Here's how the part is built. I have some questions about the finished solid (model axes, mm). Round coordinates to 2 decimals unless told otherwise and drop trailing zeros. Write each loop counter-clockwise with the first axis right and the second up, starting at its lowest first coordinate (ties: lowest second). Pieces come first, ordered by that corner, then holes. Notation, with made-up numbers: M 59,-8 L 108,-8 A25 cw 108,14 Z; hole C 7,67 d4. An arc over 180 degrees is marked long. Write item = value, one per line. Start each with the question number.
(1) I want a section at B-B (x = 63.5). List the corners of the cut face in (y, z) for me.
(2) Will these pins go through, and if not, where does the flat tip stop? pin 1 Ø2.5 at (x, z) = (142.5, -20) entering from +Y; pin 2 Ø1.2 at (x, y) = (-124, 1) entering from -Z.
(3) I want a section at C-C (y = 3.2). Give the number of separate pieces and of enclosed holes in the cut face, and give its area (3 significant figures).
(4) I need wall thicknesses on line 1 along X through (y, z) = (2.65, -60); line 2 along X through (y, z) = (1.3, 33); line 3 along X through (y, z) = (1.7, 187). Which ranges of each line are inside material? Lowest first, please.
(5) I want a section at A-A (x = -48). List the corners of the cut face in (y, z) for me.
```python
from build123d import *

# Parameters (mm, degrees)
SKETCH_1_W          = 300
SKETCH_1_H          = 500
EXTRUDE_1_DEPTH     = 4
SKETCH_2_R          = 2.5
CUT_EXTRUDE_5_DEPTH = 292.575033225
SKETCH_4_R          = 2
SKETCH_4_W          = 42
SKETCH_4_H          = 25
CUT_EXTRUDE_4_DEPTH = 292.575033225
SKETCH_5_R          = 2
CUT_EXTRUDE_6_DEPTH = 10
SKETCH_3_R          = 2
CUT_EXTRUDE_2_DEPTH = 292.575033225
CHAMFER_1_SIZE      = 2


with BuildPart() as part:
    # 草图1 → 凸台-拉伸1 (new body)
    with BuildSketch(Plane(origin=(0, 0, 0), x_dir=(1, 0, 0), z_dir=(0, 1, 0))):
        Rectangle(SKETCH_1_W, SKETCH_1_H)
    extrude(amount=EXTRUDE_1_DEPTH)

    # 草图2 → 切除-拉伸5 (cut, through all)
    with BuildSketch(Plane(origin=(0, 0, 0), x_dir=(1, 0, 0), z_dir=(0, 1, 0))):
        with Locations(Location((125, -180, 0), (0, 0, 270))):
            Circle(SKETCH_2_R)
        with Locations(Location((125, -120, 0), (0, 0, 270))):
            Circle(SKETCH_2_R)
        with Locations(Location((125, -60, 0), (0, 0, 270))):
            Circle(SKETCH_2_R)
        with Locations(Location((125, 0, 0), (0, 0, 270))):
            Circle(SKETCH_2_R)
        with Locations(Location((125, 60, 0), (0, 0, 270))):
            Circle(SKETCH_2_R)
        with Locations(Location((125, 120, 0), (0, 0, 270))):
            Circle(SKETCH_2_R)
        with Locations(Location((125, 180, 0), (0, 0, 270))):
            Circle(SKETCH_2_R)
        with Locations(Location((-125, 180, 0), (0, 0, 90))):
            Circle(SKETCH_2_R)
        with Locations(Location((-125, 120, 0), (0, 0, 90))):
            Circle(SKETCH_2_R)
        with Locations(Location((-125, 60, 0), (0, 0, 90))):
            Circle(SKETCH_2_R)
        with Locations(Location((-125, 0, 0), (0, 0, 90))):
            Circle(SKETCH_2_R)
        with Locations(Location((-125, -60, 0), (0, 0, 90))):
            Circle(SKETCH_2_R)
        with Locations(Location((-125, -120, 0), (0, 0, 90))):
            Circle(SKETCH_2_R)
        with Locations(Location((-125, -180, 0), (0, 0, 90))):
            Circle(SKETCH_2_R)
    extrude(amount=CUT_EXTRUDE_5_DEPTH, mode=Mode.SUBTRACT)

    # 草图4 → 切除-拉伸4 (cut, through all)
    with BuildSketch(Plane(origin=(0, 0, 0), x_dir=(1, 0, 0), z_dir=(0, 1, 0))):
        with Locations(Location((-78, 240, 0), (0, 0, 270))):
            Circle(SKETCH_4_R)
        with Locations(Location((-78, 220, 0), (0, 0, 270))):
            Circle(SKETCH_4_R)
        with Locations(Location((-36, 220, 0), (0, 0, 90))):
            Circle(SKETCH_4_R)
        with Locations(Location((-36, 240, 0), (0, 0, 90))):
            Circle(SKETCH_4_R)
        Polygon((-80, -175), (15, -175), (15, -25), (80, -25), (80, -225), (-80, -225), (-80, -203), (-150, -203), (-150, -197), (-80, -197), align=None)
        Polygon((-74, 235), (-40, 235), (-40, 210), (-28, 210), (-28, 198), (-40, 198), (-40, 155), (-74, 155), (-74, 198), (-86, 198), (-86, 210), (-74, 210), align=None)
        with Locations((129, 237.5)):
            Rectangle(SKETCH_4_W, SKETCH_4_H)
        with Locations((-129, 237.5)):
            Rectangle(SKETCH_4_W, SKETCH_4_H)
        with Locations((129, -237.5)):
            Rectangle(SKETCH_4_W, SKETCH_4_H)
        with Locations((-129, -237.5)):
            Rectangle(SKETCH_4_W, SKETCH_4_H)
    extrude(amount=CUT_EXTRUDE_4_DEPTH, mode=Mode.SUBTRACT)

    # 草图5 → 切除-拉伸6 (cut)
    with BuildSketch(Plane(origin=(0, 0, 0), x_dir=(1, 0, 0), z_dir=(0, 1, 0))):
        with Locations(Location((-40, -170, 0), (0, 0, 270))):
            Circle(SKETCH_5_R)
        with Locations(Location((-40, -230, 0), (0, 0, 270))):
            Circle(SKETCH_5_R)
    extrude(amount=CUT_EXTRUDE_6_DEPTH, mode=Mode.SUBTRACT)

    # 草图3 → 切除-拉伸2 (cut, through all)
    with BuildSketch(Plane(origin=(0, 0, 0), x_dir=(1, 0, 0), z_dir=(0, 1, 0))):
        with Locations(Location((-113, -187, 0), (0, 0, 270))):
            Circle(SKETCH_3_R)
        with Locations(Location((-87, -187, 0), (0, 0, 270))):
            Circle(SKETCH_3_R)
        with Locations(Location((-113, -213, 0), (0, 0, 270))):
            Circle(SKETCH_3_R)
        with Locations(Location((-87, -213, 0), (0, 0, 270))):
            Circle(SKETCH_3_R)
        with Locations(Location((-113, -7, 0), (0, 0, 270))):
            Circle(SKETCH_3_R)
        with Locations(Location((-113, -33, 0), (0, 0, 270))):
            Circle(SKETCH_3_R)
        with Locations(Location((-87, -7, 0), (0, 0, 270))):
            Circle(SKETCH_3_R)
        with Locations(Location((-87, -33, 0), (0, 0, 270))):
            Circle(SKETCH_3_R)
        with Locations(Location((87, -33, 0), (0, 0, 90))):
            Circle(SKETCH_3_R)
        with Locations(Location((87, -7, 0), (0, 0, 90))):
            Circle(SKETCH_3_R)
        with Locations(Location((113, -33, 0), (0, 0, 90))):
            Circle(SKETCH_3_R)
        with Locations(Location((113, -7, 0), (0, 0, 90))):
            Circle(SKETCH_3_R)
        with Locations(Location((87, -213, 0), (0, 0, 90))):
            Circle(SKETCH_3_R)
        with Locations(Location((113, -213, 0), (0, 0, 90))):
            Circle(SKETCH_3_R)
        with Locations(Location((87, -187, 0), (0, 0, 90))):
            Circle(SKETCH_3_R)
        with Locations(Location((113, -187, 0), (0, 0, 90))):
            Circle(SKETCH_3_R)
        with Locations(Location((-142.5, -160, 0), (0, 0, 270))):
            Circle(SKETCH_3_R)
        with Locations(Location((-142.5, -100, 0), (0, 0, 270))):
            Circle(SKETCH_3_R)
        with Locations(Location((-142.5, -40, 0), (0, 0, 270))):
            Circle(SKETCH_3_R)
        with Locations(Location((-142.5, 20, 0), (0, 0, 270))):
            Circle(SKETCH_3_R)
        with Locations(Location((-142.5, 80, 0), (0, 0, 270))):
            Circle(SKETCH_3_R)
        with Locations(Location((-142.5, 140, 0), (0, 0, 270))):
            Circle(SKETCH_3_R)
        with Locations(Location((-142.5, 200, 0), (0, 0, 270))):
            Circle(SKETCH_3_R)
        with Locations(Location((142.5, 200, 0), (0, 0, 90))):
            Circle(SKETCH_3_R)
        with Locations(Location((142.5, 140, 0), (0, 0, 90))):
            Circle(SKETCH_3_R)
        with Locations(Location((142.5, 80, 0), (0, 0, 90))):
            Circle(SKETCH_3_R)
        with Locations(Location((142.5, 20, 0), (0, 0, 90))):
            Circle(SKETCH_3_R)
        with Locations(Location((142.5, -40, 0), (0, 0, 90))):
            Circle(SKETCH_3_R)
        with Locations(Location((142.5, -100, 0), (0, 0, 90))):
            Circle(SKETCH_3_R)
        with Locations(Location((142.5, -160, 0), (0, 0, 90))):
            Circle(SKETCH_3_R)
        with Locations((27.5, -40)):
            Circle(SKETCH_3_R)
        with Locations(Location((27.5, 10, 0), (0, 0, 270))):
            Circle(SKETCH_3_R)
        with Locations(Location((27.5, 60, 0), (0, 0, 270))):
            Circle(SKETCH_3_R)
        with Locations(Location((27.5, 110, 0), (0, 0, 270))):
            Circle(SKETCH_3_R)
        with Locations(Location((27.5, 160, 0), (0, 0, 270))):
            Circle(SKETCH_3_R)
        with Locations(Location((27.5, 210, 0), (0, 0, 270))):
            Circle(SKETCH_3_R)
    extrude(amount=CUT_EXTRUDE_2_DEPTH, mode=Mode.SUBTRACT)

    # 倒角1
    chamfer_1_edges = [part.edges().sort_by_distance(p)[0] for p in [
        (-142.5, 4, -82),
        (-142.5, 4, -142),
        (-142.5, 4, -202),
        (142.5, 4, -138),
        (142.5, 4, -198),
        (-142.5, 4, 98),
        (-142.5, 4, 38),
        (-142.5, 4, -22),
        (142.5, 4, 162),
        (142.5, 4, 102),
        (142.5, 4, 42),
        (142.5, 4, -18),
        (142.5, 4, -78),
        (-142.5, 4, 158),
    ]]
    chamfer(chamfer_1_edges, length=CHAMFER_1_SIZE)


solid = part.part
```
Returned:
q1.outline = M 0,-250 L 4,-250 L 4,25 L 0,25 Z; M 0,225 L 4,225 L 4,250 L 0,250 Z
q2.pin_1 = through
q2.pin_2 = -225
q3.separate_pieces = 1
q3.enclosed_holes = 56
q3.area = 124,000 mm²
q4.line_1 = -150 to -127.5, -122.5 to 25.5, 29.5 to 122.5, 127.5 to 150
q4.line_2 = -150 to -115, -111 to -89, -85 to 15, 80 to 85, 89 to 111, 115 to 150
q4.line_3 = -150 to -115, -111 to -89, -85 to -80, 80 to 85, 89 to 111, 115 to 150
q5.outline = M 0,-250 L 4,-250 L 4,-235 L 0,-235 Z; M 0,-155 L 4,-155 L 4,175 L 0,175 Z; M 0,225 L 4,225 L 4,250 L 0,250 Z
